```python
from build123d import *

# Parameters (mm, degrees)
SKETCH1_R           = 1.75
BOSS_EXTRUDE1_DEPTH = 1.5
SKETCH2_R           = 1.75
CUT_EXTRUDE1_DEPTH  = 3
FILLET1_R           = 3
SKETCH4_W           = 80
SKETCH4_H           = 3.8
CUT_EXTRUDE3_DEPTH  = 1.5
SKETCH5_W           = 3.8
SKETCH5_H           = 102.45
CUT_EXTRUDE4_DEPTH  = 1.5


with BuildPart() as part:
    # Sketch1 → Boss-Extrude1 (new body)
    with BuildSketch(Plane(origin=(0, 0, 0), x_dir=(1, 0, 0), z_dir=(0, 1, 0))):
        Polygon((0, 55), (125, 55), (125, -55), (0, -55), (-86, -55), (-86, 55), align=None)
        with Locations(Location((0, 45, 0), (0, 0, 270))):
            Circle(SKETCH1_R, mode=Mode.SUBTRACT)
        with Locations(Location((22.5, 38.97114317, 0), (0, 0, 270))):
            Circle(SKETCH1_R, mode=Mode.SUBTRACT)
        with Locations(Location((38.97114317, 22.5, 0), (0, 0, 270))):
            Circle(SKETCH1_R, mode=Mode.SUBTRACT)
        with Locations(Location((45, 0, 0), (0, 0, 270))):
            Circle(SKETCH1_R, mode=Mode.SUBTRACT)
        with Locations(Location((38.97114317, -22.5, 0), (0, 0, 270))):
            Circle(SKETCH1_R, mode=Mode.SUBTRACT)
        with Locations(Location((22.5, -38.97114317, 0), (0, 0, 270))):
            Circle(SKETCH1_R, mode=Mode.SUBTRACT)
        with Locations(Location((0, -45, 0), (0, 0, 270))):
            Circle(SKETCH1_R, mode=Mode.SUBTRACT)
        with Locations(Location((-22.5, -38.97114317, 0), (0, 0, 270))):
            Circle(SKETCH1_R, mode=Mode.SUBTRACT)
        with Locations(Location((-38.97114317, -22.5, 0), (0, 0, 270))):
            Circle(SKETCH1_R, mode=Mode.SUBTRACT)
        with Locations(Location((-45, 0, 0), (0, 0, 270))):
            Circle(SKETCH1_R, mode=Mode.SUBTRACT)
        with Locations(Location((-38.97114317, 22.5, 0), (0, 0, 270))):
            Circle(SKETCH1_R, mode=Mode.SUBTRACT)
        with Locations(Location((-22.5, 38.97114317, 0), (0, 0, 270))):
            Circle(SKETCH1_R, mode=Mode.SUBTRACT)
    extrude(amount=BOSS_EXTRUDE1_DEPTH)

    # Sketch2 → Cut-Extrude1 (cut)
    with BuildSketch(Plane(origin=(0, 1.5, 0), x_dir=(1, 0, 0), z_dir=(0, 1, 0))):
        with Locations(Location((-10.5, -52, 0), (0, 0, 270))):
            Circle(SKETCH2_R)
        with Locations(Location((49.5, -52, 0), (0, 0, 270))):
            Circle(SKETCH2_R)
        with Locations(Location((109.5, -52, 0), (0, 0, 270))):
            Circle(SKETCH2_R)
        with Locations(Location((-70.5, -52, 0), (0, 0, 270))):
            Circle(SKETCH2_R)
        with Locations(Location((122, -44.5, 0), (0, 0, 270))):
            Circle(SKETCH2_R)
        with Locations(Location((122, 0, 0), (0, 0, 270))):
            Circle(SKETCH2_R)
        with Locations(Location((53, 0, 0), (0, 0, 90))):
            Circle(SKETCH2_R)
        with Locations(Location((53, -44.5, 0), (0, 0, 90))):
            Circle(SKETCH2_R)
        with Locations(Location((-53, -44.5, 0), (0, 0, 270))):
            Circle(SKETCH2_R)
        with Locations(Location((-53, 0, 0), (0, 0, 270))):
            Circle(SKETCH2_R)
        with BuildLine():
            Line((-83, -51.2), (-78, -51.2))
            ThreePointArc((-78, -51.2), (-77.2, -52), (-78, -52.8))
            Line((-78, -52.8), (-83, -52.8))
            ThreePointArc((-83, -52.8), (-83.8, -52), (-83, -51.2))
        make_face()
        with BuildLine():
            Line((-58, -51.2), (-63, -51.2))
            ThreePointArc((-63, -51.2), (-63.8, -52), (-63, -52.8))
            Line((-63, -52.8), (-58, -52.8))
            ThreePointArc((-58, -52.8), (-57.2, -52), (-58, -51.2))
        make_face()
        with BuildLine():
            Line((-23, -51.2), (-18, -51.2))
            ThreePointArc((-18, -51.2), (-17.2, -52), (-18, -52.8))
            Line((-18, -52.8), (-23, -52.8))
            ThreePointArc((-23, -52.8), (-23.8, -52), (-23, -51.2))
        make_face()
        with BuildLine():
            Line((2, -51.2), (-3, -51.2))
            ThreePointArc((-3, -51.2), (-3.8, -52), (-3, -52.8))
            Line((-3, -52.8), (2, -52.8))
            ThreePointArc((2, -52.8), (2.8, -52), (2, -51.2))
        make_face()
        with BuildLine():
            Line((37, -51.2), (42, -51.2))
            ThreePointArc((42, -51.2), (42.8, -52), (42, -52.8))
            Line((42, -52.8), (37, -52.8))
            ThreePointArc((37, -52.8), (36.2, -52), (37, -51.2))
        make_face()
        with BuildLine():
            Line((62, -51.2), (57, -51.2))
            ThreePointArc((57, -51.2), (56.2, -52), (57, -52.8))
            Line((57, -52.8), (62, -52.8))
            ThreePointArc((62, -52.8), (62.8, -52), (62, -51.2))
        make_face()
        with BuildLine():
            Line((97, -51.2), (102, -51.2))
            ThreePointArc((102, -51.2), (102.8, -52), (102, -52.8))
            Line((102, -52.8), (97, -52.8))
            ThreePointArc((97, -52.8), (96.2, -52), (97, -51.2))
        make_face()
        with BuildLine():
            Line((122, -51.2), (117, -51.2))
            ThreePointArc((117, -51.2), (116.2, -52), (117, -52.8))
            Line((117, -52.8), (122, -52.8))
            ThreePointArc((122, -52.8), (122.8, -52), (122, -51.2))
        make_face()
        with BuildLine():
            Line((122.8, -7.5), (122.8, -12.5))
            ThreePointArc((122.8, -12.5), (122, -13.3), (121.2, -12.5))
            Line((121.2, -12.5), (121.2, -7.5))
            ThreePointArc((121.2, -7.5), (122, -6.7), (122.8, -7.5))
        make_face()
        with BuildLine():
            Line((122.8, -32), (122.8, -37))
            ThreePointArc((122.8, -37), (122, -37.8), (121.2, -37))
            Line((121.2, -37), (121.2, -32))
            ThreePointArc((121.2, -32), (122, -31.2), (122.8, -32))
        make_face()
        with BuildLine():
            Line((52.2, -32), (52.2, -37))
            ThreePointArc((52.2, -37), (53, -37.8), (53.8, -37))
            Line((53.8, -37), (53.8, -32))
            ThreePointArc((53.8, -32), (53, -31.2), (52.2, -32))
        make_face()
        with BuildLine():
            Line((52.2, -7.5), (52.2, -12.5))
            ThreePointArc((52.2, -12.5), (53, -13.3), (53.8, -12.5))
            Line((53.8, -12.5), (53.8, -7.5))
            ThreePointArc((53.8, -7.5), (53, -6.7), (52.2, -7.5))
        make_face()
        with BuildLine():
            Line((-52.2, -7.5), (-52.2, -12.5))
            ThreePointArc((-52.2, -12.5), (-53, -13.3), (-53.8, -12.5))
            Line((-53.8, -12.5), (-53.8, -7.5))
            ThreePointArc((-53.8, -7.5), (-53, -6.7), (-52.2, -7.5))
        make_face()
        with BuildLine():
            Line((-52.2, -32), (-52.2, -37))
            ThreePointArc((-52.2, -37), (-53, -37.8), (-53.8, -37))
            Line((-53.8, -37), (-53.8, -32))
            ThreePointArc((-53.8, -32), (-53, -31.2), (-52.2, -32))
        make_face()
    cut_extrude1 = extrude(amount=-CUT_EXTRUDE1_DEPTH, mode=Mode.SUBTRACT)

    # Fillet1
    fillet1_edges = [part.edges().sort_by_distance(p)[0] for p in [
        (-86, 0.75, 55),
        (-86, 0.75, -55),
        (125, 0.75, -55),
        (125, 0.75, 55),
    ]]
    fillet(fillet1_edges, radius=FILLET1_R)

    # Mirror1: Cut-Extrude1 across plane
    add(cut_extrude1.mirror(Plane.XY), mode=Mode.SUBTRACT)

    # Sketch4 → Cut-Extrude3 (cut)
    with BuildSketch(Plane(origin=(0, 1.5, 0), x_dir=(1, 0, 0), z_dir=(0, 1, 0))):
        with Locations((85, -53.1)):
            Rectangle(SKETCH4_W, SKETCH4_H)
        with Locations((85, 53.1)):
            Rectangle(SKETCH4_W, SKETCH4_H)
    extrude(amount=-CUT_EXTRUDE3_DEPTH, mode=Mode.SUBTRACT)

    # Sketch5 → Cut-Extrude4 (cut)
    with BuildSketch(Plane(origin=(0, 1.5, 0), x_dir=(1, 0, 0), z_dir=(0, 1, 0))):
        with Locations((123.1, -0.025)):
            Rectangle(SKETCH5_W, SKETCH5_H)
    extrude(amount=-CUT_EXTRUDE4_DEPTH, mode=Mode.SUBTRACT)


solid = part.part
```
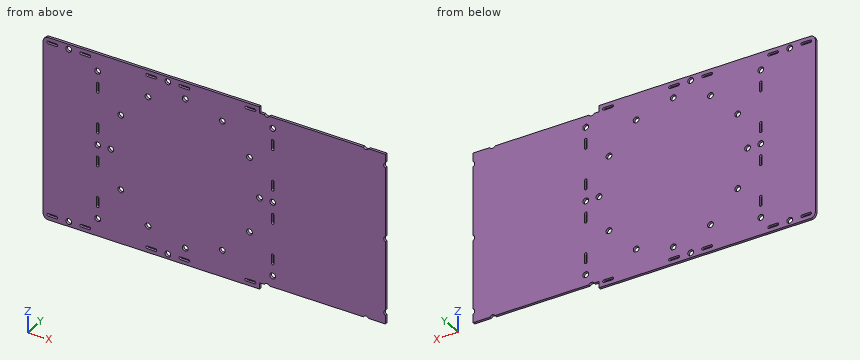
Input: part model. Units: mm. Frame: model coordinates. Coordinates: 2 decimals unless noted, no trailing zeros. Order: outer loops, then holes, each group sorted by start corner. A loop starts at its lowest first (then second) coordinate and runs counter-clockwise, first axis right, second up. Notation, with made-up numbers: (-30.75, -25) - (-13.75, -25) arc R31 ccw to (-13.75, 9) - close; hole circle Ø1 at (46.5, 88). An arc over 180 degrees is marked (long way). Put each result on its own line as item: value.
1. Line query: line 1 along Z through (x, y) = (-70.5, 0.3); line 2 along X through (y, z) = (0.65, -22.5); line 3 along X through (y, z) = (1.3, 9). Output: solid intervals per line, ascending.
Report:
line 1: z = -55 to -53.75, -50.25 to 50.25, 53.75 to 55
line 2: x = -86 to -40.72, -37.22 to 37.22, 40.72 to 121.2
line 3: x = -86 to -53.8, -52.2 to 52.2, 53.8 to 121.2
2. Cut plane B-B on y = 0.55. State how many separate pieces and enclosed holes the cut face has, then the cut area to 3 significant figures.
Report:
separate pieces: 1
enclosed holes: 40
area: 21,800 mm2
3. Contact query for a flat-ended pin moving along its axis: pin 1 Ø0.8 at (y, z) = (0.5, -52.5) entering from +X. Output: stop coordinate, or through.
Report:
pin 1: stops at x = 45
4. Cut plane A-A on x = 62.5. Return the cut outline in (y, z), then the cut area to 3 significant figures.
Report:
outline: (0, -51.2) - (1.5, -51.2) - (1.5, 51.2) - (0, 51.2) - close
area: 154 mm2
